CAD build for the part. Positions are in the model's coordinates, mm. A direction names the side the tool comes from. Round coordinates to 2 decimals unless told otherwise and drop trailing zeros. Order: outer loops, then holes, each group sorted by start corner. A loop starts at its lowest first (then second) coordinate and runs counter-clockwise, first axis right, second up. Notation, with made-up numbers: M 5,49.5 L 16,49.5 A14 ccw 16,59.5 Z; hole C 2.25,44 d4. An arc over 180 degrees is marked long. Answer as a JSON object with one key per item and string values.
```python
from build123d import *

# Parameters (mm, degrees)
SKETCH1_2_W             = 20.2
SKETCH1_2_H             = 10.6
SKETCH1_2_W_2           = 18.2
SKETCH1_2_H_2           = 8.6
BOSS_EXTRUDE1_DEPTH     = 17
SKETCH3_W               = 8.6
SKETCH3_H               = 1
BOSS_EXTRUDE2_DEPTH     = 19.2
SKETCH4_W               = 19.2
SKETCH4_H               = 9.6
CUT_EXTRUDE1_DEPTH      = 1.3
CUT_EXTRUDE2_REACH      = 22.472
SKETCH6_R               = 1.5
SKETCH8_W               = 0.4
SKETCH8_H               = 11
BOSS_EXTRUDE3_DEPTH     = 3
CUT_EXTRUDE3_DEPTH      = 27.186446876
CUT_EXTRUDE3_DEPTH_BACK = 27.186446876
SKETCH11_W              = 0.5
SKETCH11_H              = 0.6
FILLET12_R              = 0.1
FILLET13_R              = 0.1
SKETCH13_W              = 1.7
SKETCH13_H              = 1.6
CUT_EXTRUDE4_DEPTH      = 0.7


with BuildPart() as part:
    # Sketch1<2> → Boss-Extrude1 (new body)
    with BuildSketch(Plane(origin=(0, 0, 0), x_dir=(1, 0, 0), z_dir=(0, 1, 0))):
        Rectangle(SKETCH1_2_W, SKETCH1_2_H)
        Rectangle(SKETCH1_2_W_2, SKETCH1_2_H_2, mode=Mode.SUBTRACT)
    extrude(amount=BOSS_EXTRUDE1_DEPTH)

    # Sketch3 → Boss-Extrude2 (add)
    with BuildSketch(Plane(origin=(-9.1, 0, 0), x_dir=(0, 0, -1), z_dir=(1, 0, 0))):
        with Locations((0, 0.5)):
            Rectangle(SKETCH3_W, SKETCH3_H)
    extrude(amount=BOSS_EXTRUDE2_DEPTH)

    # Sketch4 → Cut-Extrude1 (cut)
    with BuildSketch(Plane(origin=(0, 17, 0), x_dir=(1, 0, 0), z_dir=(0, 1, 0))):
        Rectangle(SKETCH4_W, SKETCH4_H)
    extrude(amount=-CUT_EXTRUDE1_DEPTH, mode=Mode.SUBTRACT)

    # Sketch6 → Cut-Extrude2 (cut, up to next)
    with BuildSketch(Plane.XZ, mode=Mode.PRIVATE) as cut_extrude2_sk1:
        with Locations(Location((0, 2, 0), (0, 0, 270))):
            Circle(SKETCH6_R)
    cut_extrude2_tool1 = extrude(cut_extrude2_sk1.sketch, amount=-CUT_EXTRUDE2_REACH, mode=Mode.PRIVATE) & part.part
    add(cut_extrude2_tool1.solids().sort_by_distance((0, 0, 2))[0], mode=Mode.SUBTRACT)

    # Sketch8 → Boss-Extrude3 (add)
    with BuildSketch(Plane(origin=(-9.1, 0, 0), x_dir=(0, 0, -1), z_dir=(1, 0, 0))):
        with Locations((0.1, 6.5)):
            Rectangle(SKETCH8_W, SKETCH8_H)
    boss_extrude3 = extrude(amount=BOSS_EXTRUDE3_DEPTH)

    # Mirror1: Boss-Extrude3 across plane
    add(boss_extrude3.mirror(Plane(origin=(0, 0, 0), x_dir=(0, 0, 1), z_dir=(1, 0, 0))))

    # Sketch11 → Cut-Extrude3 (cut, two sides: drawn at the far end of the back side and taken through both)
    with BuildSketch(Plane(origin=(-9.1, 0, 0), x_dir=(0, 0, -1), z_dir=(1, 0, 0)).offset(-CUT_EXTRUDE3_DEPTH_BACK)):
        with Locations((2.55, 2.3)):
            Rectangle(SKETCH11_W, SKETCH11_H)
    extrude(amount=CUT_EXTRUDE3_DEPTH + CUT_EXTRUDE3_DEPTH_BACK, mode=Mode.SUBTRACT)

    # Fillet12
    fillet12_edges = [part.edges().sort_by_distance(p)[0] for p in [
        (10.1, 8.5, 5.3),
        (-10.1, 8.5, 5.3),
        (-10.1, 8.5, -5.3),
        (10.1, 8.5, -5.3),
    ]]
    fillet(fillet12_edges, radius=FILLET12_R)

    # Fillet13
    fillet13_edges = [part.edges().sort_by_distance(p)[0] for p in [
        (0, 0, 5.3),
        (0, 0, -5.3),
        (10.1, 0, 0),
        (-10.1, 0, 0),
        (-10.070710678, 0, -5.270710678),
        (10.070710678, 0, -5.270710678),
        (10.070710678, 0, 5.270710678),
        (-10.070710678, 0, 5.270710678),
    ]]
    fillet(fillet13_edges, radius=FILLET13_R)

    # Sketch13 → Cut-Extrude4 (cut)
    with BuildSketch(Plane(origin=(-9.1, 0, 0), x_dir=(0, 0, -1), z_dir=(1, 0, 0))):
        with Locations((2.35, 2.3)):
            Rectangle(SKETCH13_W, SKETCH13_H)
    cut_extrude4 = extrude(amount=-CUT_EXTRUDE4_DEPTH, mode=Mode.SUBTRACT)

    # Mirror2: Cut-Extrude4 across plane
    add(cut_extrude4.mirror(Plane(origin=(0, 0, 0), x_dir=(0, 0, 1), z_dir=(1, 0, 0))), mode=Mode.SUBTRACT)


solid = part.part
```
Item 1: Saw through at D-D on x = -3.5. List the corners of the cut face in (y, z), and give its area (3 significant figures).
Worked answers:
{"outline": "M 0,-5.2 A0.1 ccw 0.1,-5.3 L 17,-5.3 L 17,-4.8 L 15.7,-4.8 L 15.7,-4.3 L 1,-4.3 L 1,4.3 L 15.7,4.3 L 15.7,4.8 L 17,4.8 L 17,5.3 L 0.1,5.3 A0.1 ccw 0,5.2 Z", "area": "41.3 mm2"}
Item 2: Wall check: line 1 along Z through (x, y) = (-2.75, 16); line 2 along X through (y, z) = (0.4, 2); line 3 along Z through (x, y) = (9, 4.75). Give the ranges that are in metal, low to high. Write a range as [from, to].
Worked answers:
{"line 1": "z = [-5.3, -4.8], [4.8, 5.3]", "line 2": "x = [-10.1, -1.5], [1.5, 10.1]", "line 3": "z = [-5.3, -4.3], [-0.3, 0.1], [4.3, 5.3]"}
Item 3: Saw through at B-B on z = 2. List the corners of the cut face in (x, y), and give its area (3 significant figures).
Worked answers:
{"outline": "M -10.1,0.1 A0.1 ccw -10,0 L -1.5,0 L -1.5,1 L -9.1,1 L -9.1,15.7 L -9.6,15.7 L -9.6,17 L -10.1,17 Z; M 1.5,0 L 10,0 A0.1 ccw 10.1,0.1 L 10.1,17 L 9.6,17 L 9.6,15.7 L 9.1,15.7 L 9.1,1 L 1.5,1 Z", "area": "47.9 mm2"}
Item 4: Two-plate mould, pull along X, no slides. Class faces 4 (the flat face through (10.1, 8, 0)), 5 (the flat face through (0, 8, -5.3)), 6 (the flat face through (-0.8, 15.7, 4.6)): released by +X, released by -X, zero draft, split by the parting line, or undercut.
Worked answers:
{"face 4": "released by +X", "face 5": "zero draft", "face 6": "undercut"}
Item 5: Drop flat-ended pins along their axis: pin 1 Ø1 at (x, z) = (7.5, 2) entering from +Y; pin 2 Ø5 at (x, z) = (4.5, -0.5) entering from +Y. Give the stop position or say it passes through.
Worked answers:
{"pin 1": "stops at y = 1", "pin 2": "stops at y = 12"}
Item 6: Saw through at A-A on x = 0. List the corners of the cut face in (y, z), and give its area (3 significant figures).
Worked answers:
{"outline": "M 0,-5.2 A0.1 ccw 0.1,-5.3 L 17,-5.3 L 17,-4.8 L 15.7,-4.8 L 15.7,-4.3 L 1,-4.3 L 1,0.5 L 0,0.5 Z; M 0,3.5 L 1,3.5 L 1,4.3 L 15.7,4.3 L 15.7,4.8 L 17,4.8 L 17,5.3 L 0.1,5.3 A0.1 ccw 0,5.2 Z", "area": "38.3 mm2"}
Item 7: Saw through at C-C on x = -8.5. List the corners of the cut face in (y, z).
Worked answers:
{"outline": "M 0,-5.2 A0.1 ccw 0.1,-5.3 L 17,-5.3 L 17,-4.8 L 15.7,-4.8 L 15.7,-4.3 L 1,-4.3 L 1,-0.3 L 12,-0.3 L 12,0.1 L 1,0.1 L 1,4.3 L 15.7,4.3 L 15.7,4.8 L 17,4.8 L 17,5.3 L 0.1,5.3 A0.1 ccw 0,5.2 Z"}
Item 8: 3-axis set-ups, long thin cutter, end or side, ignore diameter. For faces 1 (the flat face through (-1, 17, 5)), 2 (the flat face through (-9.1, 8, 1)), 3 (the flat face through (9.8, 2, -2)): which of +Z, -Z, +X, -X, +Y, -Y reach the whole face in a straight line?
Worked answers:
{"face 1": "+Z, -Z, +X, -X, +Y", "face 2": "+Y", "face 3": "none"}
